Autodesk Inventor part; units mm, degrees
ref_plane "YZ Plane" through (0, 0, 0) normal (1, 0, 0) x (0, 1, 0)
ref_plane "XZ Plane" through (0, 0, 0) normal (0, 1, 0) x (-1, 0, 0)
ref_plane "XY Plane" through (0, 0, 0) normal (0, 0, 1) x (1, 0, 0)
sketch "草图2" plane through (0, 0, 0) normal (0, 0, 1) x (1, 0, 0)
  line L0 (-6.9375, 0) -> (-4.4, 0)
  arc A0 (-0.9227, 6.8759) -> (-6.9375, 0) centre (0, 0) ccw
  line L1 (-0.9227, 6.8759) -> (-0.9227, 4.3022)
  arc A1 (0.9227, 4.3022) -> (-0.9227, 4.3022) centre (0, 0) ccw
  line L2 (0.9227, 4.3022) -> (0.9227, 6.8759)
  arc A2 (6.9375, 0) -> (0.9227, 6.8759) centre (0, 0) ccw
  line L3 (4.4, 0) -> (6.9375, 0)
  arc A3 (6.7982, -6.6) -> (-6.7982, -6.6) centre (0, 0) ccw
  line L4 (0, -3.55) -> (0, 5.55)
  line L5 (-4.4, 0) -> (-4.4, -6.6)
  line L6 (-4.4, -6.6) -> (-6.7982, -6.6)
  line L7 (4.4, 0) -> (4.4, -6.6)
  line L8 (4.4, -6.6) -> (6.7982, -6.6)
  dimension "d29" = 18.95
  dimension "d33" = 13.875
  dimension "d39" = 0.9227
  dimension "d40" = 4.4
  dimension "d41" = 6.6
extrude "拉伸1" add sketch "草图2" along normal blind 0.9
fillet "圆角1" radius 1.2687 4 edges at (-6.9375, 0, 0.45) (-0.9227, 6.8759, 0.45) (0.9227, 6.8759, 0.45) (6.9375, 0, 0.45)
fillet "圆角2" radius 2.9333 2 edges at (-4.4, -6.6, 0.45) (4.4, -6.6, 0.45)
equation "\"d29\" = l2"
equation "\"d33\" = 0.5 * Diam2 + 0.5 * l2"
equation "\"d39\" = -0.0909091 * Diam2 + 0.0909091 * l2"
equation "\"d40\" = 0.5 * Diam2"
equation "\"d41\" = 0.75 * Diam2"
equation "\"d20\" = t1"
equation "\"d22\" = -0.125 * Diam2 + 0.125 * l2"
equation "\"d42\" = 0.333333 * Diam2"
equation "\"l2\" = 18.95"
equation "\"t1\" = 0.9"
equation "\"Diam2\" = 8.8"
equation "\"sd\" = 11"
equation "\"TEMPLATE\" = 1.2345"
properties part number "ASME B27.8M - 3EM1-11" material "钢，软"
Could you check a few things on this model? Use its own coordinates, in mm. A direction names the side the tool comes from. Coordinates: 2 decimals unless noted, no trailing zeros. Order: outer loops, then holes, each group sorted by start corner. A loop starts at its lowest first (then second) coordinate and runs counter-clockwise, first axis right, second up. Notation, with made-up numbers: (25, -22.75) -> (73, -22.75) arc R24 cw to (73, 6.25) -> close; hole circle Ø3 at (53.5, -10). An arc over 180 degrees is marked (long way). One line per item, written item: value. Start each with the question number.
1) Imagine slicing it at C-C on x = 6.5. List the corners of the cut face in (y, z) for me, plus the area to 3 significant figures.
2) If I drill on L1, parallel to X at y = 5.5, z = 0.75; L2, parallel to X at y = 5, z = 0.15; L3, parallel to X at y = -4.5, z = 0.1, over which ranges is the centre line in solid material (lowest first)? Write a range as [from, to].
3) We'd pull the mould along X, two halves only. Please class faces 1 (the flat face through (0, 5, 0.9)), 2 (the cylindrical face through (-0.31, 9.47, 0.44)), 3 (the flat face through (-4.4, -1.8, 0.4)): +X half, -X half, draft (parallel to the pull), parting line (faces both ways), or undercut.
4) Which directions (+Z, -Z, +X, -X, +Y, -Y) give clear straight access to the entire face, cutting with the end or side of a thin tool? Please do faces 4 (the flat face through (4.4, -1.8, 0.4)), 5 (the flat face through (0, 5, 0)), 6 (the flat face through (-5, 0, 0.4)).
5) Imagine slicing it at D-D on y = 5.5. List the corners of the cut face in (x, z) for me, plus the area to 3 significant figures.
6) Imagine slicing it at A-A on y = -0.25. List the corners of the cut face in (x, z) for me, plus the area to 3 significant figures.
7) I'm going to push flat-ended pins straight in: pin 1 (0.5 mm diameter, centred on y = -1, z = 0.5, fed in from +X); pin 2 (0.5 mm diameter, centred on y = -2, z = 0.5, fed in from -X). Where does each tip first touch, or does it pass through?
8) Imagine slicing it at B-B on z = 0.7. List the corners of the cut face in (x, y) for me (3 decimals), plus the area to 3 significant figures.
Answer list:
1. outline: (-6.53, 0) -> (0.46, 0) -> (0.46, 0.9) -> (-6.53, 0.9) -> close; (2.42, 0) -> (6.89, 0) -> (6.89, 0.9) -> (2.42, 0.9) -> close
1. area: 10.3 mm2
2. L1: x = [-7.72, -4.23], [-0.95, 0.95], [4.23, 7.72]
2. L2: x = [-8.05, -4.81], [-0.92, 0.92], [4.81, 8.05]
2. L3: x = [-8.34, -4.51], [4.51, 8.34]
3. face 1: draft
3. face 2: parting line
3. face 3: undercut
4. face 4: +Z, -Z, -Y
4. face 5: -Z, +X, -X, +Y, -Y
4. face 6: +Z, -Z
5. outline: (-7.72, 0) -> (-4.23, 0) -> (-4.23, 0.9) -> (-7.72, 0.9) -> close; (-0.95, 0) -> (0.95, 0) -> (0.95, 0.9) -> (-0.95, 0.9) -> close; (4.23, 0) -> (7.72, 0) -> (7.72, 0.9) -> (4.23, 0.9) -> close
5. area: 7.99 mm2
6. outline: (-9.47, 0) -> (-4.4, 0) -> (-4.4, 0.9) -> (-9.47, 0.9) -> close; (4.4, 0) -> (9.47, 0) -> (9.47, 0.9) -> (4.4, 0.9) -> close
6. area: 9.13 mm2
7. pin 1: stops at x = 9.45
7. pin 2: stops at x = -9.31
8. outline: (-6.798, -6.6) arc R2.933 ccw to (-4.4, -3.716) -> (-4.4, 0) -> (-5.525, 0) arc R1.269 cw to (-6.762, 1.553) arc R6.937 cw to (-2.682, 6.398) arc R1.269 cw to (-0.923, 5.228) -> (-0.923, 4.302) arc R4.4 cw to (0.923, 4.302) -> (0.923, 5.228) arc R1.269 cw to (2.682, 6.398) arc R6.938 cw to (6.762, 1.553) arc R1.269 cw to (5.525, 0) -> (4.4, 0) -> (4.4, -3.716) arc R2.933 ccw to (6.798, -6.6) arc R9.475 ccw (long way) to start
8. area: 125 mm2
